The model under review builds one solid part; all positions refer to its coordinate system, in mm. Round coordinates to 2 decimals unless told otherwise and drop trailing zeros. Order: outer loops, then holes, each group sorted by start corner. A loop starts at its lowest first (then second) coordinate and runs counter-clockwise, first axis right, second up. Notation, with made-up numbers: M 62,-4 L 120,-4 A7 cw 120,5 Z; hole C 56.5,35.5 d2. An arc over 180 degrees is marked long. Answer as CSV lines item,"result". Start each with the question number.
from build123d import *

# Parameters (mm, degrees)
SHEET_EXTRUDE_1_1_DEPTH = 84
THICKEN_1_T2            = 0.1


with BuildPart() as body_1:
    # Sheet Extrude 1: a surface, the sketch's curves swept straight by 84 mm
    with BuildLine(Plane.XY, mode=Mode.PRIVATE) as sheet_extrude_1_1_path:
        Line((1.799379952, 0), (1.799379952, 0.3))
        ThreePointArc((1.799379952, 0.3), (1.049689976, 0.638210804), (0.3, 0.3))
        Line((0.3, 0.3), (0.3, 0))
        Line((0.3, 0), (0, 0))
        Line((0, 0), (0, 12.1))
        ThreePointArc((0, 12.1), (0.585786438, 13.514213562), (2, 14.1))
    sheet_extrude_1_1 = Shell.extrude(sheet_extrude_1_1_path.wire(), (0 * SHEET_EXTRUDE_1_1_DEPTH, 0 * SHEET_EXTRUDE_1_1_DEPTH, 1 * SHEET_EXTRUDE_1_1_DEPTH))
    add(Solid.thicken(sheet_extrude_1_1, -THICKEN_1_T2))


solid = body_1.part
Item 1: Consider section B-B (x = 0.8). State the section outline as (y, z) points, and give its area (3 significant figures).
Item 2: Consider section A-A (z = 10). State the section outline as (x, y) points, and give its area (3 significant figures).
Item 3: Wall thickness on probe 1 along Y at (x, z) = (0.25, 51): over which ranges is the line inside the solid? List them lowest first. Write a range as [from, to].
Item 4: Consider section C-C (y = 3). State the section outline as (x, z) points.
Reported:
1,outline,"M 0.61,0 L 0.71,0 L 0.71,84 L 0.61,84 Z; M 13.57,0 L 13.7,0 L 13.7,84 L 13.57,84 Z"
1,area,"19.3 mm²"
2,outline,"M 0,0 L 0.3,0 L 0.3,0.3 A1 cw 1.8,0.3 L 1.8,0 L 1.9,0 L 1.9,0.34 A1.1 ccw 0.2,0.34 L 0.2,0.1 L 0.1,0.1 L 0.1,12.1 A1.9 cw 2,14 L 2,14.1 A2 ccw 0,12.1 Z"
2,area,"1.77 mm²"
3,probe 1,"y = [0, 0.39], [12.84, 13.07]"
4,outline,"M 0,0 L 0.1,0 L 0.1,84 L 0,84 Z"
